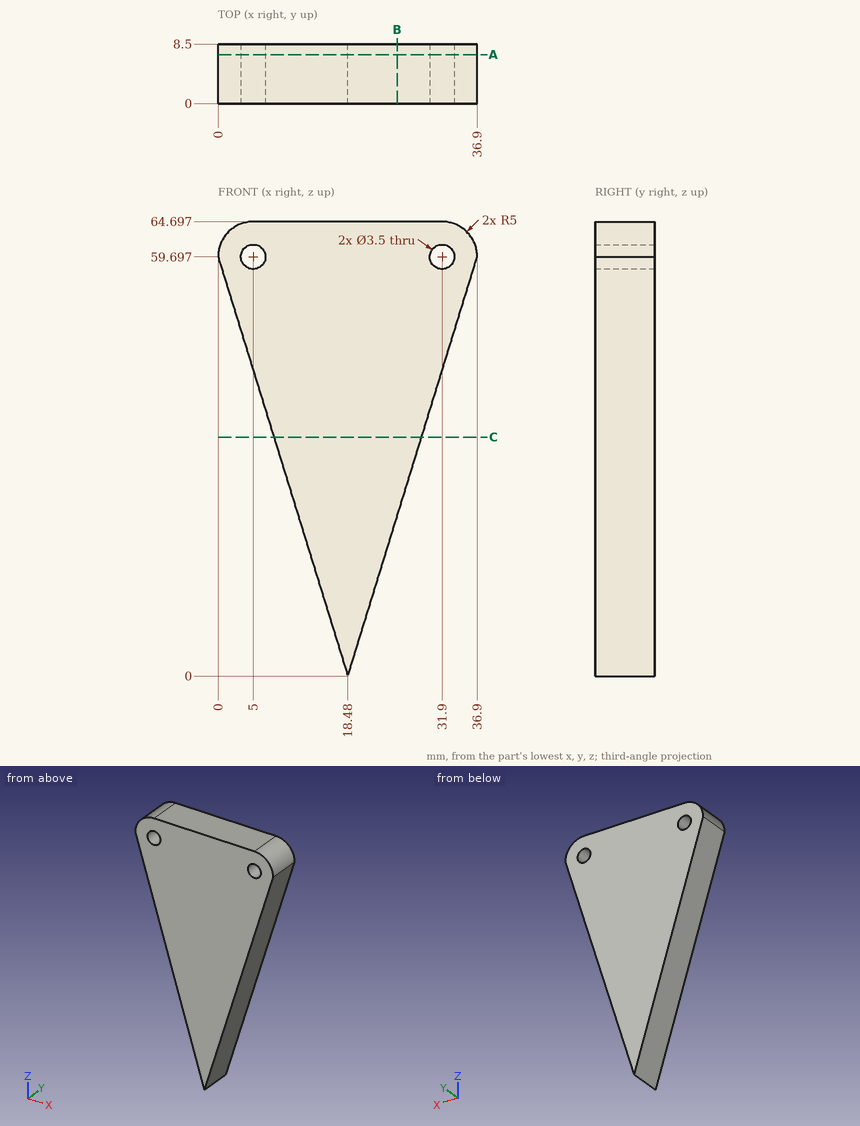
Design review of the part shown in the three views and the two pictorial views. Dimensions are in mm from the part's minimum x, y and z. Round coordinates to 2 decimals unless told otherwise and drop trailing zeros. Write each loop counter-clockwise with the first axis right and the second up, starting at its lowest first coordinate (ties: lowest second). Pieces come first, ordered by that corner, then holes.
Item 1: We need section C-C on z = 34. Write out the cut boundary in (x, y) (1 decimal), and give its area (3 significant figures).
Item 2: For probe 1 along X at (y, z) = (4.75, 59.5); probe 2 along X at (y, z) = (8, 10) (1 decimal); probe 3 along X at (y, z) = (1.25, 30), list the stretches that pass through material, from the lowest coordinate up.
Item 3: We need section A-A on y = 7. Write out the cut boundary in (x, z), and give its area (3 significant figures).
Item 4: We need section B-B on x = 25.5. Write out the cut boundary in (y, z).
Item 5: Clearance check with flat-ended pins moving along their axes: pin 1 Ø3 at (x, z) = (31.9, 59.7) entering from +Y; pin 2 Ø5 at (x, z) = (13, 21.5) entering from -Y; pin 3 Ø2 at (y, z) = (5.5, 54.5) entering from +X (3 decimals); pin 4 Ø1.5 at (y, z) = (5.5, 26.5) entering from +X. State where each tip first meets the part, or that it passes through.
Returned:
1. outline: (8, 0) - (29, 0) - (29, 8.5) - (8, 8.5) - close
1. area: 179 mm2
2. probe 1: x = 0.06 to 3.26, 6.74 to 30.16, 33.64 to 36.84
2. probe 2: x = 15.4 to 21.6
2. probe 3: x = 9.19 to 27.74
3. outline: (0, 59.7) - (18.48, 0) - (36.9, 59.7) arc R5 ccw to (31.9, 64.7) - (5, 64.7) arc R5 ccw to start; hole circle Ø3.5 at (5, 59.7); hole circle Ø3.5 at (31.9, 59.7)
3. area: 1,260 mm2
4. outline: (0, 22.75) - (8.5, 22.75) - (8.5, 64.7) - (0, 64.7) - close
5. pin 1: passes through
5. pin 2: stops at y = 0
5. pin 3: stops at x = 35.605
5. pin 4: stops at x = 26.89
